CAD build for the part. Positions are in the model's coordinates, mm. Face numbers are marked on the shaded views. A direction names the side the tool comes from. Give positions to 0.01 mm unless a question says otherwise; leave off trailing zeros. Write each loop counter-clockwise with the first axis right and the second up, starting at its lowest first coordinate (ties: lowest second). Pieces come first, ordered by that corner, then holes. Notation, with made-up numbers: (50.5, -3) - (81.5, -3) arc R10 ccw to (81.5, 13) - close; hole circle Ø5 at (3.25, 27.25). An arc over 180 degrees is marked (long way). Put each result on its own line as item: value. Start each with the question number.
1. Drop flat-ended pins along their axis: pin 1 (12 mm diameter, centred on x = -17, y = 38.5, fed in from -Z); pin 2 (10 mm diameter, centred on x = -55, z = -17.5, fed in from -Y). Give the stop position or say it passes through.
2. Cut at A-A on x = 92.5. List the corners of the cut face in (y, z), and give its area (3 significant figures).
3. Cut at C-C on z = -11. List the corners of the cut face in (x, y), and give its area (3 significant figures).
4. Cut at B-B on y = 23. List the corners of the cut face in (x, z).
5. Wall check: line 1 (Z direction, x = 189, y = 46); line 2 (Y direction, x = 85, z = -10.5). Give the ranges that are in metal, low to high.
6. Tool access for the marked faces 1 and 2: list every direction of +Z, -Z, +X, -X, +Y, -Y with a clear straight run to the whole face (end or side of a thin tool).
from build123d import *

# Parameters (mm, degrees)
SKETCH1_W           = 448
SKETCH1_H           = 70
BASE_FLANGE1_DEPTH  = 4
SKETCH6_W           = 448
SKETCH6_H           = 4
BOSS_EXTRUDE1_DEPTH = 20


# Sheet-metal steps are written as plain solids
with BuildPart() as part:
    # Sketch1 → Base-Flange1 (new body)
    with BuildSketch(Plane.XY):
        with Locations((0, 35)):
            Rectangle(SKETCH1_W, SKETCH1_H)
    extrude(amount=-BASE_FLANGE1_DEPTH)

    # Sketch6 → Boss-Extrude1 (add)
    with BuildSketch(Plane(origin=(0, 0, -4), x_dir=(-1, 0, 0), z_dir=(0, 0, -1))):
        with Locations((0, 68)):
            Rectangle(SKETCH6_W, SKETCH6_H)
    extrude(amount=BOSS_EXTRUDE1_DEPTH)


solid = part.part
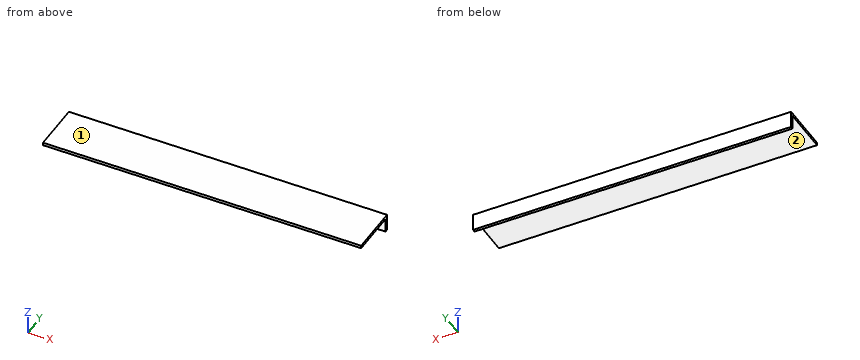
Report:
1. pin 1: stops at z = -4
1. pin 2: stops at y = 66
2. outline: (0, -4) - (66, -4) - (66, -24) - (70, -24) - (70, 0) - (0, 0) - close
2. area: 360 mm²
3. outline: (-224, 66) - (224, 66) - (224, 70) - (-224, 70) - close
3. area: 1,790 mm²
4. outline: (-224, -4) - (224, -4) - (224, 0) - (-224, 0) - close
5. line 1: z = -4 to 0
5. line 2: y = 66 to 70
6. face 1: +Z, +X, -X, +Y, -Y
6. face 2: -Z, +X, -X, -Y
